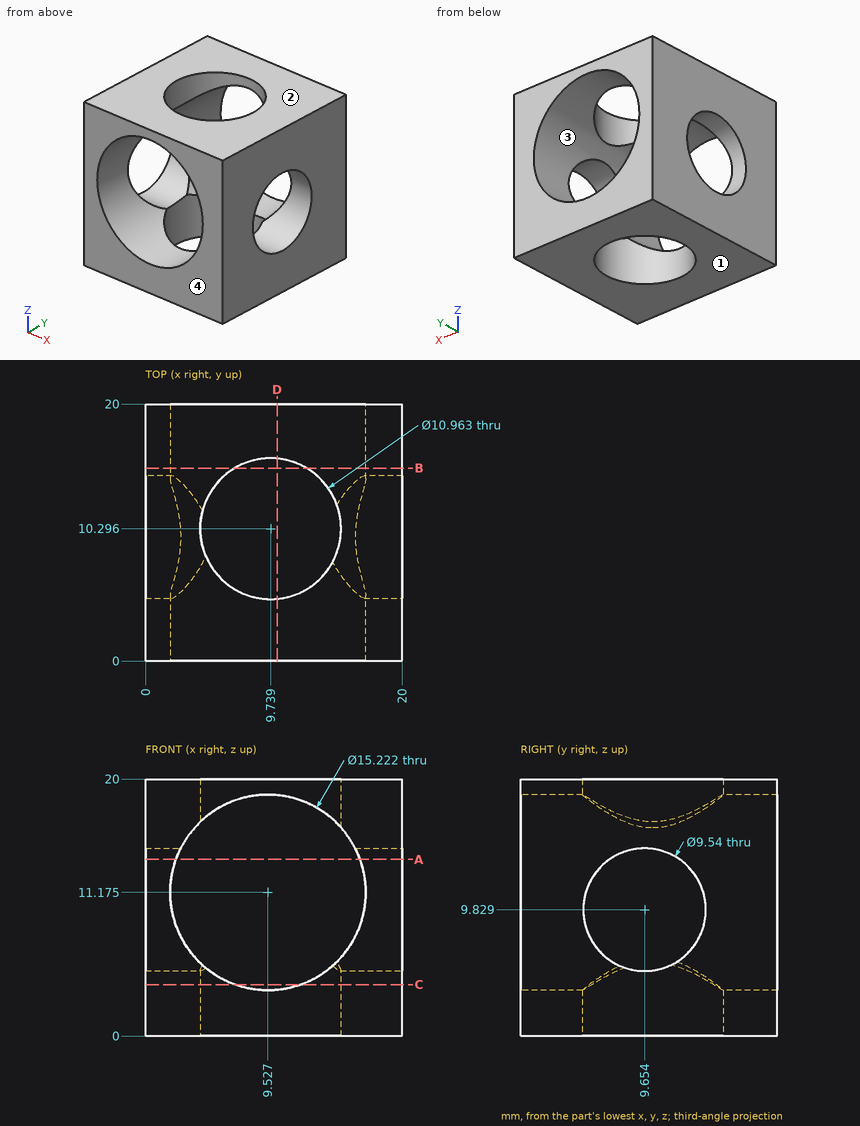
Input: dimensioned drawing with shaded views. Units: mm. Origin: part minimum x, y, z. Give positions to 0.01 mm unless a question says otherwise; leave off trailing zeros. Write each loop counter-clockwise with the first axis right and the second up, starting at its lowest first coordinate (ties: lowest second). Pieces come first, ordered by that corner, then holes.
1. Section query B-B, the plane y = 15. Return loops of the section in (x, z) (1 decimal), then the cut area to 3 significant figures.
2. Line query: probe 1 along Z at (x, y) = (16.5, 9.25); probe 2 along Y at (x, z) = (19, 7.25) (1 decimal); probe 3 along Y at (x, z) = (17.25, 12) (1 decimal). Output: solid intervals per line, ascending.
3. Draft query along Z for the marked faces 1, 2, 3 and 4. Return one class per face: released by +Z, released by -Z, zero draft, split by the parting line, or undercut.
4. Section query A-A, the plane z = 13.75. Return loops of the section in (x, y) (1 decimal).
5. Section query C-C, the plane z = 4. Return loops of the section in (x, y) (1 decimal).
6. Section query D-D, the plane x = 10.25. Return loops of the section in (y, z).
Computed:
1. outline: (0, 0) - (6.9, 0) - (6.9, 4) arc R7.6 cw to (6.9, 18.3) - (6.9, 20) - (0, 20) - close; (12.6, 0) - (20, 0) - (20, 20) - (12.6, 20) - (12.6, 18.2) arc R7.6 cw to (12.6, 4.2) - close
1. area: 189 mm2
2. probe 1: z = 0 to 5.08, 14.58 to 20
2. probe 2: y = 0 to 5.6, 13.7 to 20
2. probe 3: y = 0 to 5.4, 13.9 to 20
3. face 1: released by -Z
3. face 2: released by +Z
3. face 3: undercut
3. face 4: zero draft
4. outline: (0, 0) - (2.4, 0) - (2.4, 6.9) - (0, 6.9) - close; (0, 12.4) - (2.4, 12.4) - (2.4, 20) - (0, 20) - close; (16.7, 0) - (20, 0) - (20, 6.9) - (16.7, 6.9) - close; (16.7, 12.4) - (20, 12.4) - (20, 20) - (16.7, 20) - close
5. outline: (0, 0) - (7, 0) - (7, 5.6) arc R5.5 cw to (7, 15) - (7, 20) - (0, 20) - close; (12.1, 0) - (20, 0) - (20, 20) - (12.1, 20) - (12.1, 15.3) arc R5.5 cw to (12.1, 5.3) - close
6. outline: (0, 0) - (4.84, 0) - (4.84, 3.6) - (0, 3.6) - close; (0, 18.75) - (4.84, 18.75) - (4.84, 20) - (0, 20) - close; (15.75, 0) - (20, 0) - (20, 3.6) - (15.75, 3.6) - close; (15.75, 18.75) - (20, 18.75) - (20, 20) - (15.75, 20) - close
